Verification items for the finished model (mm, model axes). A direction names the side the tool comes from. Round coordinates to 2 decimals unless told otherwise and drop trailing zeros. Loops run counter-clockwise (first coordinate to the right, second up) from the corner with the lowest first, then second, coordinate; pieces in that order, holes last. Notation, with made-up numbers: (-7, 49.25) -> (40, 49.25) arc R20 cw to (40, 54.25) -> close; hole circle Ø7 at (67.25, 51). An arc over 180 degrees is marked (long way). Use CSV: the item, a comma, the result in double quotes. Start each with the question number.
```python
from build123d import *

# Parameters (mm, degrees)
SKIZZE1_W                       = 50
SKIZZE1_H                       = 60
SKIZZE1_R                       = 1.25
AUFSATZ_LINEAR_AUSTRAGEN1_DEPTH = 10
SKIZZE2_R                       = 1.5
AUFSATZ_LINEAR_AUSTRAGEN2_DEPTH = 4
SKIZZE3_W                       = 50
SKIZZE3_H                       = 10
SKIZZE3_R                       = 1.25
AUFSATZ_LINEAR_AUSTRAGEN3_DEPTH = 2.5


with BuildPart() as part:
    # Skizze1 → Aufsatz-Linear austragen1 (new body)
    with BuildSketch(Plane.XY):
        with Locations((-25, 30)):
            Rectangle(SKIZZE1_W, SKIZZE1_H)
        with Locations((-45, 57.05)):
            Circle(SKIZZE1_R, mode=Mode.SUBTRACT)
        with Locations((-5, 57.05)):
            Circle(SKIZZE1_R, mode=Mode.SUBTRACT)
        with Locations((-45, 2.95)):
            Circle(SKIZZE1_R, mode=Mode.SUBTRACT)
        with Locations((-5, 2.95)):
            Circle(SKIZZE1_R, mode=Mode.SUBTRACT)
    extrude(amount=AUFSATZ_LINEAR_AUSTRAGEN1_DEPTH)

    # Skizze2 → Aufsatz-Linear austragen2 (add)
    with BuildSketch(Plane.XY.offset(10)):
        with Locations((-25, 30)):
            Circle(SKIZZE2_R)
    extrude(amount=AUFSATZ_LINEAR_AUSTRAGEN2_DEPTH)

    # Skizze3 → Aufsatz-Linear austragen3 (add)
    with BuildSketch(Plane.XY.offset(10)):
        with Locations((-25, 55)):
            Rectangle(SKIZZE3_W, SKIZZE3_H)
        with Locations((-45, 57.05)):
            Circle(SKIZZE3_R, mode=Mode.SUBTRACT)
        with Locations((-5, 57.05)):
            Circle(SKIZZE3_R, mode=Mode.SUBTRACT)
        with Locations((-25, 5)):
            Rectangle(SKIZZE3_W, SKIZZE3_H)
        with Locations((-45, 2.95)):
            Circle(SKIZZE3_R, mode=Mode.SUBTRACT)
        with Locations((-5, 2.95)):
            Circle(SKIZZE3_R, mode=Mode.SUBTRACT)
    extrude(amount=AUFSATZ_LINEAR_AUSTRAGEN3_DEPTH)


solid = part.part
```
Q1. Cross-section at D-D (x = -25). Record the boundary of the cut face in (y, z).
Q2. Depth check by flat-ended pin: pin 1 Ø2 at (x, y) = (-45, 57.05) entering from -Z; pin 2 Ø3 at (x, y) = (-5, 57.05) entering from +Z. Enter the tip coordinate at first touch or a pass-through.
Q3. Thickness scan on L1, parallel to Y at x = -5, z = 3.25; L2, parallel to Y at x = -23, z = 11.5; L3, parallel to Z at x = -24, y = 24.5. Record the ranges inside material, lowest first. Write a range as from..to.
Q4. Cross-section at C-C (x = -5). Record the boundary of the cut face in (y, z).
Q5. Cross-section at B-B (y = 57.05). Record the boundary of the cut face in (x, z).
Q6. Cross-section at A-A (z = 10.75). Record the boundary of the cut face in (x, y), and give its area (3 significant figures).
Q7. Tool access check on faces 1 (the face through (0, 30, 5)), 2 (the face through (-26.11, 31.01, 11.97)), 3 (the face through (-25, 50, 11)). Record the directions out of +Z, -Z, +X, -X, +Y, -Y that give a thin tool (end or side, any length) a straight path to the whole face; none if there is none.
Q8. Release check for a two-part mould opening along Y. For faces 4 (the face through (-25, 5, 12.5)), 5 (the face through (-46, 2.2, 6.2)), 6 (the face through (-25, 0, 6)) record: +Y half, -Y half, draft (parallel to the pull), parting line (faces both ways), or undercut.
Answer list:
1,outline,"(0, 0) -> (60, 0) -> (60, 12.5) -> (50, 12.5) -> (50, 10) -> (31.5, 10) -> (31.5, 14) -> (28.5, 14) -> (28.5, 10) -> (10, 10) -> (10, 12.5) -> (0, 12.5) -> close"
2,pin 1,"passes through"
2,pin 2,"stops at z = 12.5"
3,L1,"y = 0..1.7, 4.2..55.8, 58.3..60"
3,L2,"y = 0..10, 50..60"
3,L3,"z = 0..10"
4,outline,"(0, 0) -> (1.7, 0) -> (1.7, 12.5) -> (0, 12.5) -> close; (4.2, 0) -> (55.8, 0) -> (55.8, 12.5) -> (50, 12.5) -> (50, 10) -> (10, 10) -> (10, 12.5) -> (4.2, 12.5) -> close; (58.3, 0) -> (60, 0) -> (60, 12.5) -> (58.3, 12.5) -> close"
5,outline,"(-50, 0) -> (-46.25, 0) -> (-46.25, 12.5) -> (-50, 12.5) -> close; (-43.75, 0) -> (-6.25, 0) -> (-6.25, 12.5) -> (-43.75, 12.5) -> close; (-3.75, 0) -> (0, 0) -> (0, 12.5) -> (-3.75, 12.5) -> close"
6,outline,"(-50, 0) -> (0, 0) -> (0, 10) -> (-50, 10) -> close; (-50, 50) -> (0, 50) -> (0, 60) -> (-50, 60) -> close; circle Ø3 at (-25, 30); hole circle Ø2.5 at (-45, 2.95); hole circle Ø2.5 at (-45, 57.05); hole circle Ø2.5 at (-5, 2.95); hole circle Ø2.5 at (-5, 57.05)"
6,area,"987 mm2"
7,face 1,"+Z, -Z, +X, +Y, -Y"
7,face 2,"+Z"
7,face 3,"+Z, +X, -X"
8,face 4,"draft"
8,face 5,"undercut"
8,face 6,"-Y half"
